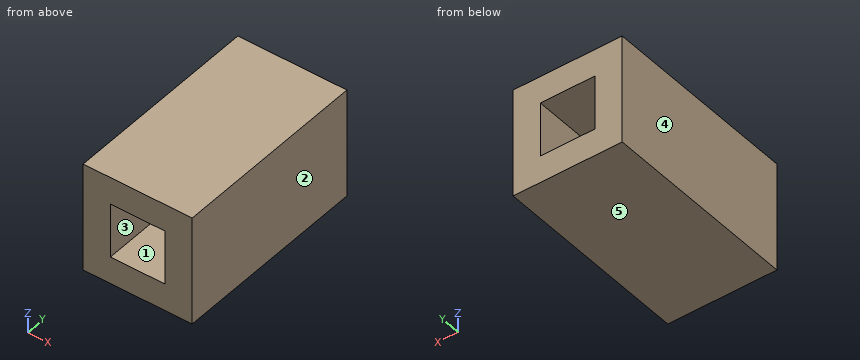
Autodesk Inventor part; units mm, degrees
ref_plane "YZ Plane" through (0, 0, 0) normal (1, 0, 0) x (0, 1, 0)
ref_plane "XZ Plane" through (0, 0, 0) normal (0, 1, 0) x (-1, 0, 0)
ref_plane "XY Plane" through (0, 0, 0) normal (0, 0, 1) x (1, 0, 0)
sketch "Sketch1" plane through (0, 0, 0) normal (0, 0, 1) x (1, 0, 0)
  line L0 (-38.1, -69.85) -> (38.1, -69.85)
  line L1 (38.1, -69.85) -> (38.1, 69.85)
  line L2 (38.1, 69.85) -> (-38.1, 69.85)
  line L3 (-38.1, 69.85) -> (-38.1, -69.85)
  line L4 (19.05, 69.85) -> (19.05, -69.85)
  line L5 (-19.05, 69.85) -> (-19.05, -69.85)
  line L6 (-19.05, 69.85) -> (19.05, 69.85)
  point P0 (0, 0)
  point P1 (38.1, 6.35)
  point P2 (-38.1, -57.15)
  point P3 (38.1, 57.15)
  point P4 (-38.1, -6.35)
  point P5 (0, 69.85)
  dimension "d0" = 139.7
  dimension "d1" = 76.2
  dimension "d13" = 38.1
extrude "Extrusion1" add sketch "Sketch1" along normal blind 38.1 contours L3 L2 L5 L0 | L4 L2 L1 L0
sketch "Sketch2" plane through (0, 0, 38.1) normal (0, 0, 1) x (1, 0, 0)
  line L0 (-38.1, 69.85) -> (-38.1, -69.85)
  line L1 (38.1, -69.85) -> (-38.1, -69.85)
  line L2 (-38.1, -69.85) -> (-38.1, 69.85)
  line L3 (-38.1, 69.85) -> (38.1, 69.85)
  line L4 (38.1, 69.85) -> (38.1, -69.85)
  line L5 (38.1, -69.85) -> (-38.1, 69.85) construction
  line L6 (-38.1, -69.85) -> (38.1, 69.85) construction
  point P0 (0, 0)
  point P1 (-38.1, 0)
extrude "Extrusion2" add sketch "Sketch2" along normal blind 19.05
sketch "Sketch3" plane through (0, 0, 0) normal (0, 0, -1) x (-1, 0, 0)
  line L0 (38.1, 69.85) -> (38.1, -69.85)
  line L1 (-38.1, -69.85) -> (38.1, -69.85)
  line L2 (38.1, -69.85) -> (38.1, 69.85)
  line L3 (38.1, 69.85) -> (-38.1, 69.85)
  line L4 (-38.1, 69.85) -> (-38.1, -69.85)
  line L5 (-38.1, -69.85) -> (38.1, 69.85) construction
  line L6 (38.1, -69.85) -> (-38.1, 69.85) construction
  point P0 (0, 0)
  point P1 (38.1, 0)
extrude "Extrusion3" add sketch "Sketch3" along normal blind 19.05
properties part number "hollow monitor support (for assembly)"
CAD build for the part. Positions are in the model's coordinates, mm. Face numbers are marked on the shaded views. A direction names the side the tool comes from. Coordinates: 2 decimals unless noted, no trailing zeros. Write each loop counter-clockwise with the first axis right and the second up, starting at its lowest first coordinate (ties: lowest second). Pieces come first, ordered by that corner, then holes. Notation, with made-up numbers: M 3.25,-11.5 L 43.25,-11.5 A10 cw 43.25,2.5 Z; hole C 36,29.25 d3. An arc over 180 degrees is marked long. Answer as a JSON object with one key per item and string values. Group by question number.
1) Tool access for the marked faces 1 and 2: list every direction of +Z, -Z, +X, -X, +Y, -Y with a clear straight run to the whole face (end or side of a thin tool).
2) Wall check: line 1 (Z direction, x = 12.5, y = 32); line 2 (X direction, y = 1.5, z = 33.5). Give the ranges that are in metal, low to high. Write a range as from..to.
3) Saw through at B-B (x = 9.5). Write the cut outline in (y, z).
4) Saw through at C-C (y = -53.5). Write the cut outline in (x, z).
5) Mould opens along Z. For the marked faces 3, 4 and 5 say: +Z half, -Z half, draft (parallel to the pull), parting line (faces both ways), or undercut.
6) Saw through at A-A (z = 12). Write the cut outline in (x, y).
Values follow:
{
 "1": {"face 1": "+Y, -Y", "face 2": "+Z, -Z, +X, +Y, -Y"},
 "2": {"line 1": "z = -19.05..0, 38.1..57.15", "line 2": "x = -38.1..-19.05, 19.05..38.1"},
 "3": {"outline": "M -69.85,-19.05 L 69.85,-19.05 L 69.85,0 L -69.85,0 Z; M -69.85,38.1 L 69.85,38.1 L 69.85,57.15 L -69.85,57.15 Z"},
 "4": {"outline": "M -38.1,-19.05 L 38.1,-19.05 L 38.1,57.15 L -38.1,57.15 Z; hole M -19.05,0 L 19.05,0 L 19.05,38.1 L -19.05,38.1 Z"},
 "5": {"face 3": "undercut", "face 4": "draft", "face 5": "-Z half"},
 "6": {"outline": "M -38.1,-69.85 L -19.05,-69.85 L -19.05,69.85 L -38.1,69.85 Z; M 19.05,-69.85 L 38.1,-69.85 L 38.1,69.85 L 19.05,69.85 Z"}
}
